CAD build for the part. Positions are in the model's coordinates, mm. A direction names the side the tool comes from. Round coordinates to 2 decimals unless told otherwise and drop trailing zeros. Loops run counter-clockwise (first coordinate to the right, second up) from the corner with the lowest first, then second, coordinate; pieces in that order, holes last.
from build123d import *

# Parameters (mm, degrees)
SKETCH1_R               = 5.75
SKETCH1_R_2             = 4.7
BOSS_EXTRUDE1_DEPTH     = 10
CUT_EXTRUDE1_DEPTH      = 13.888948755
CUT_EXTRUDE1_DEPTH_BACK = 13.888948755
SKETCH2_R               = 2.3
SKETCH3_R               = 5.75
BOSS_EXTRUDE2_DEPTH     = 9
BOSS_EXTRUDE3_START     = 0.5
SKETCH4_R               = 4.7
BOSS_EXTRUDE3_DEPTH     = 0.5
CUT_EXTRUDE2_DEPTH      = 21.667002833
CUT_EXTRUDE2_DEPTH_BACK = 4.5
SKETCH5_R               = 2.4


with BuildPart() as part:
    # Sketch1 → Boss-Extrude1 (new body)
    with BuildSketch(Plane(origin=(0, 0, 0), x_dir=(1, 0, 0), z_dir=(0, 1, 0))):
        with Locations(Location((0, 0, 0), (0, 0, 270))):
            Circle(SKETCH1_R)
        with Locations(Location((0, 0, 0), (0, 0, 270))):
            Circle(SKETCH1_R_2, mode=Mode.SUBTRACT)
    extrude(amount=BOSS_EXTRUDE1_DEPTH)

    # Sketch2 → Cut-Extrude1 (cut, two sides: drawn at the far end of the back side and taken through both)
    with BuildSketch(Plane(origin=(0, 0, 0), x_dir=(0, 0, -1), z_dir=(1, 0, 0)).offset(-CUT_EXTRUDE1_DEPTH_BACK)):
        with Locations((0, 4.3)):
            Circle(SKETCH2_R)
    extrude(amount=CUT_EXTRUDE1_DEPTH + CUT_EXTRUDE1_DEPTH_BACK, mode=Mode.SUBTRACT)

    # Sketch3 → Boss-Extrude2 (add)
    with BuildSketch(Plane(origin=(0, 10, 0), x_dir=(1, 0, 0), z_dir=(0, 1, 0))):
        with Locations(Location((0, 0, 0), (0, 0, 270))):
            Circle(SKETCH3_R)
    extrude(amount=BOSS_EXTRUDE2_DEPTH)

    # Sketch4 → Boss-Extrude3 (add)
    with BuildSketch(Plane.XZ.offset(-10).offset(BOSS_EXTRUDE3_START)):
        with Locations(Location((0, 0, 0), (0, 0, 270))):
            Circle(SKETCH4_R)
    extrude(amount=-BOSS_EXTRUDE3_DEPTH)

    # Sketch5 → Cut-Extrude2 (cut, two sides: drawn at the far end of the back side and taken through both)
    with BuildSketch(Plane(origin=(0, 19, 0), x_dir=(1, 0, 0), z_dir=(0, 1, 0)).offset(-CUT_EXTRUDE2_DEPTH_BACK)):
        with Locations(Location((0, 0, 0), (0, 0, 90))):
            Circle(SKETCH5_R)
    extrude(amount=CUT_EXTRUDE2_DEPTH + CUT_EXTRUDE2_DEPTH_BACK, mode=Mode.SUBTRACT)


solid = part.part
Item 1: Cut at B-B (x = 0). List the corners of the cut face in (y, z).
Verdict:
outline: (0, -5.75) - (19, -5.75) - (19, -2.4) - (14.5, -2.4) - (14.5, 2.4) - (19, 2.4) - (19, 5.75) - (0, 5.75) - (0, 4.7) - (9.5, 4.7) - (9.5, -4.7) - (0, -4.7) - close
Item 2: 3-axis set-ups, long thin cutter, end or side, ignore diameter. For faces 1 (the cylindrical face through (-4.937, 6.239, -1.236)), 2 (the cylindrical face through (3.96, 4.68, 2.53)), 3 (the flat face through (0, 14.5, 0)): which of +Z, -Z, +X, -X, +Y, -Y reach the whole face in a straight line?
Verdict:
face 1: +X, -X
face 2: -Y
face 3: +Y
Item 3: Wall check: L1, parallel to Y at x = 5.05, z = 0; L2, parallel to X at y = 17.55, z = 0; L3, parallel to Y at x = -1.5, z = -1. Give the ranges that are in metal, low to high.
Verdict:
L1: y = 0 to 2, 6.6 to 19
L2: x = -5.75 to -2.4, 2.4 to 5.75
L3: y = 9.5 to 14.5
Item 4: Cut at C-C (y = 6). List the corners of the cut face in (x, z).
Verdict:
outline: (-5.54, -1.55) arc R5.75 ccw to (5.54, -1.55) - (4.44, -1.55) arc R4.7 cw to (-4.44, -1.55) - close; (-5.54, 1.55) - (-4.44, 1.55) arc R4.7 cw to (4.44, 1.55) - (5.54, 1.55) arc R5.75 ccw to start
Item 5: Cut at D-D (z = 3). List the corners of the cut face in (x, y).
Verdict:
outline: (-4.91, 0) - (-3.62, 0) - (-3.62, 9.5) - (3.62, 9.5) - (3.62, 0) - (4.91, 0) - (4.91, 19) - (-4.91, 19) - close
Item 6: Cut at A-A (z = 0). List the corners of the cut face in (x, y).
Verdict:
outline: (-5.75, 0) - (-4.7, 0) - (-4.7, 2) - (-5.75, 2) - close; (-5.75, 6.6) - (-4.7, 6.6) - (-4.7, 9.5) - (4.7, 9.5) - (4.7, 6.6) - (5.75, 6.6) - (5.75, 19) - (2.4, 19) - (2.4, 14.5) - (-2.4, 14.5) - (-2.4, 19) - (-5.75, 19) - close; (4.7, 0) - (5.75, 0) - (5.75, 2) - (4.7, 2) - close
Item 7: Mould opens along X. For faces 4 (the flat face through (0, 0, -5)), 5 (the cylindrical face through (-2.024, 16.718, -1.29)), 6 (the cylindrical face through (1.727, 9.367, 5.484)) say: released by +X, released by -X, zero draft, split by the parting line, or undercut.
Verdict:
face 4: zero draft
face 5: undercut
face 6: split by the parting line
Item 8: Flat gauge pins, fed straight in: P1, Ø3, axis at y = 4.3, z = 0, coming from the -X side; P2, Ø5, axis at x = 4, y = 13, coming from the -Z side; P3, Ø6, axis at x = 0, z = 0, coming from the -Y side; P4, Ø1.5, axis at y = 2, z = 4.5, coming from the +X side. Where does each tip first touch, or does it go through?
Verdict:
P1: passes through
P2: stops at z = -5.55
P3: stops at y = 9.5
P4: stops at x = 4.36
